Autodesk Inventor part; units mm, degrees
ref_plane "YZ Plane" through (0, 0, 0) normal (1, 0, 0) x (0, 1, 0)
ref_plane "XZ Plane" through (0, 0, 0) normal (0, 1, 0) x (-1, 0, 0)
ref_plane "XY Plane" through (0, 0, 0) normal (0, 0, 1) x (1, 0, 0)
sketch "Sketch1" plane through (0, 0, 0) normal (0, 0, 1) x (1, 0, 0)
  line L0 (-29.0928, 7.1512) -> (47.1072, 7.1512)
  line L1 (47.1072, 7.1512) -> (47.1072, 83.3512)
  line L2 (47.1072, 83.3512) -> (-29.0928, 83.3512)
  line L3 (-29.0928, 83.3512) -> (-29.0928, 7.1512)
  line L4 (-54.4928, 7.1512) -> (97.9072, 7.1512)
  line L5 (97.9072, 7.1512) -> (97.9072, -43.6488)
  line L6 (97.9072, -43.6488) -> (-54.4928, -43.6488)
  line L7 (-54.4928, -43.6488) -> (-54.4928, 7.1512)
  circle A0 centre (-48.1428, 0.8012) radius 3.175
  circle A1 centre (47.1072, -37.2988) radius 3.175
  line L8 (-46.9636, 3.7491) -> (48.2864, -34.3509)
  line L9 (-49.322, -2.1467) -> (45.928, -40.2467)
  circle A2 centre (-3.6928, 0.8012) radius 3.175
  line L10 (-4.872, -2.1467) -> (90.378, -40.2467)
  line L11 (-2.5136, 3.7491) -> (92.7364, -34.3509)
  circle A3 centre (91.5572, -37.2988) radius 3.175
  point P0 (0, 0)
  point P1 (-29.0928, 7.1512)
  dimension "d0" = 76.2
  dimension "d1" = 76.2
  dimension "d2" = 152.4
  dimension "d3" = 50.8
  dimension "d4" = 25.4
  dimension "d5" = 6.35
  dimension "d6" = 6.35
  dimension "d7" = 6.35
  dimension "d8" = 6.35
  dimension "d9" = 6.35
  dimension "d10" = 6.35
  dimension "d11" = 6.35
  dimension "d12" = 6.35
extrude "Extrusion1" add sketch "Sketch1" along normal blind 6.35
chamfer "Chamfer1" distance 6.35 angle 45 1 edges at (9.0072, 83.3512, 6.35)
properties part number "Tall Wall Lift"
CAD build for the part. Positions are in the model's coordinates, mm. A direction names the side the tool comes from. Give positions to 0.01 mm unless a question says otherwise; leave off trailing zeros. Order: outer loops, then holes, each group sorted by start corner. A loop starts at its lowest first (then second) coordinate and runs counter-clockwise, first axis right, second up. Notation, with made-up numbers: (69, -7.75) - (109, -7.75) arc R15 cw to (109, 21.25) - close; hole circle Ø6 at (40, 67.25). An arc over 180 degrees is marked (long way). Answer in a Markdown table with one row per item.
1. Probe probe 1 along Y at (x, z) = (4, 6); probe 2 along X at (y, z) = (24.5, 4); probe 3 along Y at (x, z) = (15.5, 6). List the from-to ranges inside material, lowest first. Write a range as [from, to].
Data:
| item | result |
|---|---|
| probe 1 | y = [-43.65, -23.48], [-16.64, -5.7], [1.14, 77.35] |
| probe 2 | x = [-29.09, 47.11] |
| probe 3 | y = [-43.65, -28.08], [-21.24, -10.3], [-3.46, 77.35] |
2. Saw through at C-C, the plane z = 4. Give the cut face in (x, y) (3 decimals).
Data:
| item | result |
|---|---|
| outline | (-54.493, -43.649) - (97.907, -43.649) - (97.907, 7.151) - (47.107, 7.151) - (47.107, 79.352) - (-29.093, 79.352) - (-29.093, 7.151) - (-54.493, 7.151) - close; hole (-49.322, -2.147) - (45.928, -40.247) arc R3.175 ccw to (48.286, -34.351) - (-46.964, 3.749) arc R3.175 ccw to start; hole (-4.872, -2.147) - (90.378, -40.247) arc R3.175 ccw to (92.736, -34.351) - (-2.514, 3.749) arc R3.175 ccw to start |
3. Saw through at B-B, the plane y = -6. Give the cut face in (x, z).
Data:
| item | result |
|---|---|
| outline | (-54.49, 0) - (-39.69, 0) - (-39.69, 6.35) - (-54.49, 6.35) - close; (-22.59, 0) - (4.76, 0) - (4.76, 6.35) - (-22.59, 6.35) - close; (21.86, 0) - (97.91, 0) - (97.91, 6.35) - (21.86, 6.35) - close |
4. Saw through at D-D, the plane x = 40. Count the separate pieces of the cut face and the enclosed holes in it, plus the area to 3 significant figures.
Data:
| item | result |
|---|---|
| separate pieces | 3 |
| enclosed holes | 0 |
| area | 699 mm² |
5. Tool access for faces 1 (the flat face through (-2.36, -20.93, 3.13)), 2 (the flat face through (47.107, 45, 3)), 3 (the flat face through (-29.093, 46, 3)): list every direction of +Z, -Z, +X, -X, +Y, -Y with a clear straight run to the whole face (end or side of a thin tool).
Data:
| item | result |
|---|---|
| face 1 | +Z, -Z |
| face 2 | +Z, -Z, +X, +Y |
| face 3 | +Z, -Z, -X, +Y |
6. Flat gauge pins, fed straight in: pin 1 (2 mm diameter, centred on y = 17.5, z = 4, fed in from +X); pin 2 (2 mm diameter, centred on y = 15, z = 5, fed in from -X); pin 3 (1.9 mm diameter, centred on x = -47, z = 4.5, fed in from +Y). Where does each tip first touch, or does it go through?
Data:
| item | result |
|---|---|
| pin 1 | stops at x = 47.11 |
| pin 2 | stops at x = -29.09 |
| pin 3 | stops at y = 7.15 |
